Check sheet for the modelled part. Datum: model origin and axes. Units: mm. A direction names the side the tool comes from. Coordinates: 2 decimals unless noted, no trailing zeros. Answer as CSV lines item,"result". Start each with the question number.
Q1. Sectioned sample at A-A, the plane z = 3.5. Count the separate pieces of the cut face and the enclosed holes in it, then the cut area to 3 significant figures.
Q2. Mould release check, pull along Y, two halves, no side actions. Record for faces 4 (the cylindrical face through (-3.096, -84.722, 3.131)), 5 (the cylindrical face through (-49.15, -12.6, 3.13)), 6 (the flat face through (104, -53.975, 3)), 7 (the flat face through (-27, 1.3, 3.1)): pulls with the +Y half, pulls with the -Y half, needs draft (parallel to the pull), parting line crosses it, or undercut.
Q3. Depth check by flat-ended pin: pin 1 Ø1 at (x, z) = (1, 4) entering from -Y; pin 2 Ø1.5 at (x, z) = (121, 1) entering from -Y (3 decimals); pin 3 Ø3 at (x, z) = (59, 1.5) entering from +Y. Enter the tip coordinate at first touch or a pass-through.
Q4. Thickness scan on line 1 along X through (y, z) = (-33, 4.25); line 2 along Y through (x, z) = (89.5, 2.25) (1 decimal); line 3 along Y through (x, z) = (34.5, 4) (3 decimals). Record the ranges inside material, lowest first. Write a range as from..to.
Q5. Access from +Z, -Z, +X, -X, +Y, -Y to the whole of each face (thin tool, end or side, straight path). Record for faces 1 (the cylindrical face through (16.2, -60.5, 3.1)), 2 (the flat face through (-49.72, -36.15, 3.13)), 3 (the flat face through (102.03, 8.84, 3.13)).
from build123d import *

# Parameters (mm, degrees)
MODEL_R             = 2.413
MODEL_R_2           = 12.7
MODEL_R_3           = 14.281149998
MODEL_R_4           = 3.302
MODEL_R_5           = 2.5527
MODEL_R_6           = 6.00075
MODEL_R_7           = 1.6
MODEL_R_8           = 6.599999999
BOSS_EXTRUDE2_DEPTH = 6.35
BOSS_EXTRUDE3_DEPTH = 6.35
CUT_EXTRUDE2_DEPTH  = 7.35
SKETCH3_R           = 1.75
BOSS_EXTRUDE4_DEPTH = 6.35
SKETCH3_6_R         = 1.75
CUT_EXTRUDE3_DEPTH  = 7.35
BOSS_EXTRUDE5_DEPTH = 6.35
SKETCH9_R           = 5.9944
CUT_EXTRUDE4_DEPTH  = 7.35


with BuildPart() as part:
    # Model → Boss-Extrude2 (new body)
    with BuildSketch(Plane.XY):
        with BuildLine():
            Line((33.194381935, -53.975), (176.626960261, -53.975))
            ThreePointArc((176.626960261, -53.975), (179.801405862, -42.211824955), (182.193350463, -30.264942807))
            ThreePointArc((182.193350463, -30.264942807), (183.829791454, 17.804254832), (172.999114376, 64.665989059))
            ThreePointArc((172.999114376, 64.665989059), (172.041022004, 67.851130989), (171.507342233, 71.134156425))
            Line((171.507342233, 71.134156425), (168.283057515, 104.748950069))
            ThreePointArc((168.283057515, 104.748950069), (153.768177108, 120.335666132), (134.949478429, 110.361496948))
            Line((134.949478429, 110.361496948), (120.644399952, 79.107921201))
            ThreePointArc((120.644399952, 79.107921201), (116.145567058, 72.378282822), (109.757890395, 67.405847105))
            Line((109.757890395, 67.405847105), (31.721738278, 24.629886736))
            ThreePointArc((31.721738278, 24.629886736), (20.873181942, 21.53956394), (9.756276385, 23.451547307))
            ThreePointArc((9.756276385, 23.451547307), (-9.646239085, 23.497022608), (-23.420042255, 9.831664186))
            Line((-23.420042255, 9.831664186), (-52.812443226, -60.184078795))
            ThreePointArc((-52.812443226, -60.184078795), (-31.676825474, -103.162616273), (7.980260895, -76.307737346))
            ThreePointArc((7.980260895, -76.307737346), (16.353189451, -60.360946363), (33.194381935, -53.975))
        make_face()
        with Locations((-2.78154477, -87.114522117)):
            Circle(MODEL_R, mode=Mode.SUBTRACT)
        with Locations((-44.293236039, -57.832795939)):
            Circle(MODEL_R, mode=Mode.SUBTRACT)
        with Locations((-23.537390405, -72.473659028)):
            Circle(MODEL_R_2, mode=Mode.SUBTRACT)
        with BuildLine():
            ThreePointArc((-12.841593176, -42.57947194), (-19.109154707, -40.609081586), (-12.573, -41.275))
            ThreePointArc((-12.573, -41.275), (-12.640845293, -41.940918414), (-12.841593176, -42.57947194))
        make_face(mode=Mode.SUBTRACT)
        with Locations((2e-09, -1e-09)):
            Circle(MODEL_R_3, mode=Mode.SUBTRACT)
        with Locations((9.525, -41.275)):
            Circle(MODEL_R_4, mode=Mode.SUBTRACT)
        with Locations((22.225, -41.275)):
            Circle(MODEL_R_5, mode=Mode.SUBTRACT)
        with Locations((34.925, -41.275)):
            Circle(MODEL_R_5, mode=Mode.SUBTRACT)
        with Locations((47.625, -41.275)):
            Circle(MODEL_R_5, mode=Mode.SUBTRACT)
        with Locations((60.325, -41.275)):
            Circle(MODEL_R_5, mode=Mode.SUBTRACT)
        with BuildLine():
            ThreePointArc((16.191119841, -19.570580939), (26.262071613, -14.489518063), (37.54006963, -14.270359917))
            Line((37.54006963, -14.270359917), (106.835310384, -28.641149755))
            ThreePointArc((106.835310384, -28.641149755), (109.349000903, -32.074056686), (106.19058164, -34.925))
            Line((106.19058164, -34.925), (-8.284075387, -34.925))
            ThreePointArc((-8.284075387, -34.925), (-10.484598164, -34.038738628), (-11.456624352, -31.874731974))
            Line((-11.456624352, -31.874731974), (-11.631809955, -27.418898539))
            ThreePointArc((-11.631809955, -27.418898539), (-10.39277622, -24.775805221), (-7.519343102, -24.26148139))
            ThreePointArc((-7.519343102, -24.26148139), (4.929611011, -24.917041062), (16.191119841, -19.570580939))
        make_face(mode=Mode.SUBTRACT)
        with Locations((73.025, -41.275)):
            Circle(MODEL_R_5, mode=Mode.SUBTRACT)
        with Locations((85.725, -41.275)):
            Circle(MODEL_R_5, mode=Mode.SUBTRACT)
        with Locations((98.425, -41.275)):
            Circle(MODEL_R_5, mode=Mode.SUBTRACT)
        with Locations((111.125, -41.275)):
            Circle(MODEL_R_5, mode=Mode.SUBTRACT)
        with Locations((123.825, -41.275)):
            Circle(MODEL_R_5, mode=Mode.SUBTRACT)
        with BuildLine():
            Line((150.525780255, -24.731666411), (53.587874929, -4.628204042))
            ThreePointArc((53.587874929, -4.628204042), (51.058848917, -1.430439454), (53.762941599, 1.62071667))
            Line((53.762941599, 1.62071667), (151.674333159, 16.265377518))
            ThreePointArc((151.674333159, 16.265377518), (156.599060705, 14.928824322), (158.95010909, 10.399819206))
            ThreePointArc((158.95010909, 10.399819206), (159.227492405, -4.460838665), (158.118539501, -19.282657626))
            ThreePointArc((158.118539501, -19.282657626), (155.517613032, -23.672930664), (150.525780255, -24.731666411))
        make_face(mode=Mode.SUBTRACT)
        with Locations((136.525, -41.275)):
            Circle(MODEL_R_5, mode=Mode.SUBTRACT)
        with Locations((149.225, -41.275)):
            Circle(MODEL_R_5, mode=Mode.SUBTRACT)
        with Locations((161.925, -41.275)):
            Circle(MODEL_R_5, mode=Mode.SUBTRACT)
        with Locations((174.625, -41.275)):
            Circle(MODEL_R_5, mode=Mode.SUBTRACT)
        with Locations((165.041643061, -32.828823938)):
            Circle(MODEL_R_4, mode=Mode.SUBTRACT)
        with Locations((168.275000002, -1e-09)):
            Circle(MODEL_R_4, mode=Mode.SUBTRACT)
        with BuildLine():
            Line((149.795684871, 28.825659386), (51.884293311, 14.180998537))
            ThreePointArc((51.884293311, 14.180998537), (48.40578749, 16.307419992), (49.888483051, 20.105219991))
            Line((49.888483051, 20.105219991), (136.7018524, 67.692461879))
            ThreePointArc((136.7018524, 67.692461879), (141.785005521, 68.14064733), (145.556679438, 64.703527647))
            ThreePointArc((145.556679438, 64.703527647), (150.953895829, 50.854840016), (155.036811216, 36.563377676))
            ThreePointArc((155.036811216, 36.563377676), (154.113819123, 31.54467252), (149.795684871, 28.825659386))
        make_face(mode=Mode.SUBTRACT)
        with Locations((165.041643061, 32.828823937)):
            Circle(MODEL_R_4, mode=Mode.SUBTRACT)
        with Locations((143.968148324, 91.96125582)):
            Circle(MODEL_R_6, mode=Mode.SUBTRACT)
        with Locations((155.465828334, 64.396054582)):
            Circle(MODEL_R_4, mode=Mode.SUBTRACT)
        with Locations((161.105196874, 87.885715063)):
            Circle(MODEL_R_6, mode=Mode.SUBTRACT)
        with Locations((138.411127855, 104.180489712)):
            Circle(MODEL_R_7, mode=Mode.SUBTRACT)
        with Locations((150.86241233, 103.077985772)):
            Circle(MODEL_R_8, mode=Mode.SUBTRACT)
        with Locations((151.96491627, 115.529270247)):
            Circle(MODEL_R_7, mode=Mode.SUBTRACT)
        with Locations((163.313696806, 101.975481832)):
            Circle(MODEL_R_7, mode=Mode.SUBTRACT)
    extrude(amount=BOSS_EXTRUDE2_DEPTH)

    # Sketch2 → Boss-Extrude3 (add, through all)
    with BuildSketch(Plane.XY.offset(6.35)):
        with BuildLine():
            Line((143.625048634, 85.970322406), (149.20311028, 89.027968606))
            ThreePointArc((149.20311028, 89.027968606), (146.8525684, 86.699210458), (143.625048634, 85.970322406))
        make_face()
        with BuildLine():
            ThreePointArc((164.878362916, 83.219644063), (162.13420828, 88.447058862), (159.224374167, 93.584092596))
            ThreePointArc((159.224374167, 93.584092596), (155.837304584, 85.011987277), (164.878362916, 83.219644063))
        make_face()
    extrude(amount=-BOSS_EXTRUDE3_DEPTH)

    # Sketch2<3> → Cut-Extrude2 (cut, through all)
    with BuildSketch(Plane.XY.offset(6.35)):
        with BuildLine():
            ThreePointArc((159.224374167, 93.584092596), (159.015682677, 93.938258333), (158.80620341, 94.291958693))
            Line((158.80620341, 94.291958693), (149.20311028, 89.027968606))
            Line((149.20311028, 89.027968606), (143.625048634, 85.970322406))
            Line((143.625048634, 85.970322406), (109.757890395, 67.405847105))
            ThreePointArc((109.757890395, 67.405847105), (116.145567058, 72.378282822), (120.644399952, 79.107921201))
            Line((120.644399952, 79.107921201), (134.949478429, 110.361496948))
            ThreePointArc((134.949478429, 110.361496948), (153.768177108, 120.335666132), (168.283057515, 104.748950069))
            Line((168.283057515, 104.748950069), (171.507342233, 71.134156425))
            ThreePointArc((171.507342233, 71.134156425), (172.041022004, 67.851130989), (172.999114376, 64.665989059))
            ThreePointArc((172.999114376, 64.665989059), (166.739844557, 79.424227745), (159.224374167, 93.584092596))
        make_face()
    extrude(amount=-CUT_EXTRUDE2_DEPTH, mode=Mode.SUBTRACT)

    # Sketch3 → Boss-Extrude4 (add, through all)
    with BuildSketch(Plane(origin=(0, 0, 0), x_dir=(-1, 0, 0), z_dir=(0, 0, -1))):
        with Locations((24.263890272, -19.571729998)):
            Circle(SKETCH3_R)
        with BuildLine():
            Line((47.569931866, -41.013247954), (51.934565947, -31.139666326))
            ThreePointArc((51.934565947, -31.139666326), (48.962006062, -12.385946654), (30.645740354, -7.380696976))
            Line((30.645740354, -7.380696976), (45.859161931, -43.620642669))
            ThreePointArc((45.859161931, -43.620642669), (46.821980785, -42.387435085), (47.569931866, -41.013247954))
        make_face()
        with Locations((40.421189912, -12.399445261)):
            Circle(SKETCH3_R, mode=Mode.SUBTRACT)
        with Locations((47.593474649, -28.556744901)):
            Circle(SKETCH3_R, mode=Mode.SUBTRACT)
    extrude(amount=-BOSS_EXTRUDE4_DEPTH)

    # Sketch3<6> → Cut-Extrude3 (cut, through all)
    with BuildSketch(Plane(origin=(0, 0, 0), x_dir=(-1, 0, 0), z_dir=(0, 0, -1))):
        with Locations((24.263890272, -19.571729998)):
            Circle(SKETCH3_6_R)
    extrude(amount=-CUT_EXTRUDE3_DEPTH, mode=Mode.SUBTRACT)

    # Sketch8 → Boss-Extrude5 (add, through all)
    with BuildSketch(Plane(origin=(0, 0, 0), x_dir=(-1, 0, 0), z_dir=(0, 0, -1))):
        with BuildLine():
            Line((-158.80620341, 94.291958693), (-146.170088384, 87.365400413))
            ThreePointArc((-146.170088384, 87.365400413), (-162.606044593, 102.518063532), (-166.242121917, 80.460801739))
            ThreePointArc((-166.242121917, 80.460801739), (-162.671228787, 87.455446032), (-158.80620341, 94.291958693))
        make_face()
    extrude(amount=-BOSS_EXTRUDE5_DEPTH)

    # Sketch9 → Cut-Extrude4 (cut, through all)
    with BuildSketch(Plane(origin=(0, 0, 0), x_dir=(-1, 0, 0), z_dir=(0, 0, -1))):
        with Locations((-158.474943349, 90.50873372)):
            Circle(SKETCH9_R)
    extrude(amount=-CUT_EXTRUDE4_DEPTH, mode=Mode.SUBTRACT)


solid = part.part
Output:
1,separate pieces,"1"
1,enclosed holes,"30"
1,area,"17,300 mm^2"
2,face 4,"undercut"
2,face 5,"undercut"
2,face 6,"pulls with the -Y half"
2,face 7,"pulls with the +Y half"
3,pin 1,"stops at y = -93.22"
3,pin 2,"stops at y = -53.975"
3,pin 3,"stops at y = 40.4"
4,line 1,"x = -51.11..-11.2, 109.11..161.74, 168.34..181.72"
4,line 2,"y = -54..-34.9, -25..-12.1, 7..19.8, 41.8..56.3"
4,line 3,"y = -53.975..-43.792, -38.758..-34.925, -13.83..26.153"
5,face 1,"+Z, -Z, +X, -Y"
5,face 2,"+Z, -Z, -X"
5,face 3,"+Z, -Z"
